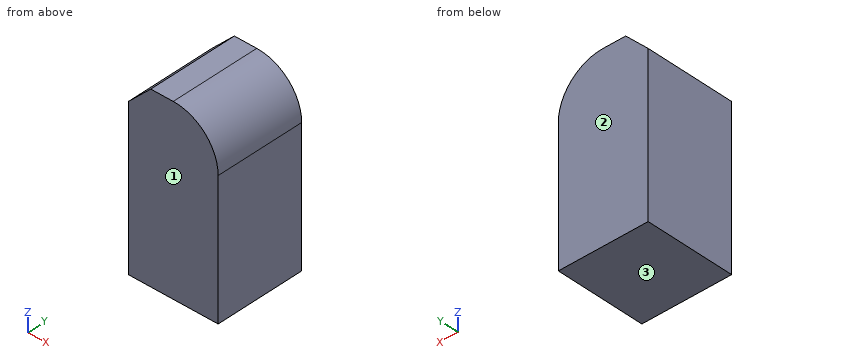
```python
from build123d import *

# Parameters (mm, degrees)
SKETCH2_W           = 20
SKETCH2_H           = 40
BOSS_EXTRUDE1_DEPTH = 20
FILLET1_R           = 10
CHAMFER1_SIZE       = 5


with BuildPart() as part:
    # Sketch2 → Boss-Extrude1 (new body)
    with BuildSketch(Plane(origin=(0, 0, 0), x_dir=(1, 0, 0), z_dir=(0, 1, 0))):
        with Locations((10, 20)):
            Rectangle(SKETCH2_W, SKETCH2_H)
    extrude(amount=BOSS_EXTRUDE1_DEPTH)

    # Fillet1
    fillet1_edges = [part.edges().sort_by_distance(p)[0] for p in [
        (20, 10, 0),
    ]]
    fillet(fillet1_edges, radius=FILLET1_R)

    # Chamfer1
    chamfer1_edges = [part.edges().sort_by_distance(p)[0] for p in [
        (0, 10, 0),
    ]]
    chamfer(chamfer1_edges, length=CHAMFER1_SIZE)


solid = part.part
```
Geometry: final body of the model. Coordinates: model frame, mm. Face numbers are marked on the shaded views. Give positions to 0.01 mm unless a question says otherwise; leave off trailing zeros. Write each loop counter-clockwise with the first axis right and the second up, starting at its lowest first coordinate (ties: lowest second). Pieces come first, ordered by that corner, then holes.
1. Section query A-A, the plane y = 18.75. Return loops of the section in (x, z), then the cut area to 3 significant figures.
2. Line query: probe 1 along Z at (x, y) = (4.5, 3.5); probe 2 along Z at (x, y) = (18.5, 13.25); probe 3 along X at (y, z) = (4, -5). Output: solid intervals per line, ascending.
3. Pin query (flat end, axial travel): P1, Ø4, axis at x = 16.5, y = 9, coming from the +Z side. Return the tip coordinate at first contact, or that it passes through.
4. Draft query along Y for the marked faces 1, 2 and 3. Return one class per face: released by +Y, released by -Y, zero draft, split by the parting line, or undercut.
5. Section query C-C, the plane z = -7. Return loops of the section in (x, y), then the cut area to 3 significant figures.
6. Section query B-B, the plane x = 16.25. Return loops of the section in (y, z).
Computed:
1. outline: (0, -40) - (20, -40) - (20, -10) arc R10 ccw to (10, 0) - (5, 0) - (0, -5) - close
1. area: 766 mm2
2. probe 1: z = -40 to -0.5
2. probe 2: z = -40 to -4.73
2. probe 3: x = 0 to 18.66
3. P1: stops at z = -1.07
4. face 1: released by -Y
4. face 2: released by +Y
4. face 3: zero draft
5. outline: (0, 0) - (19.54, 0) - (19.54, 20) - (0, 20) - close
5. area: 391 mm2
6. outline: (0, -40) - (20, -40) - (20, -2.19) - (0, -2.19) - close
